Read the model definition and answer for the solid it produces. Units are mm, in the model's axes. A direction names the side the tool comes from. Coordinates: 2 decimals unless noted, no trailing zeros. Write each loop counter-clockwise with the first axis right and the second up, starting at its lowest first coordinate (ties: lowest second). Pieces come first, ordered by that corner, then holes.
1) Each of these flat-tipped pins is pushed along its axis until it touches: pin 1 Ø3 at (y, z) = (18.5, -111) entering from +X; pin 2 Ø4 at (y, z) = (13, -108) entering from -X; pin 3 Ø2 at (x, y) = (-32, 19) entering from -Z; pin 4 Ø5 at (x, z) = (-35.5, -108.5) entering from -Y. Where does it stop, or does it pass through?
2) Determine the mould class of faces 3 (the face through (-33.47, 0.246, -111.096)), 4 (the face through (-29.46, 0.74, -110.49)), 5 (the face through (-35, 1.5, -112)), 6 (the face through (-34.12, 11.87, -110.91)) for opening direction Z: +Z half, -Z half, draft (parallel to the pull), parting line (faces both ways), or undercut.
3) The part is cut by section A-A (y = 13). Determine the outline of the cut face in (x, z).
4) Find the intervals of material crossed by line 1 (Y direction, x = -30, z = -110.5); line 2 (Z direction, x = -34.25, y = 8.5); line 3 (Z direction, x = -32.75, y = 1.25), in increasing order.
5) Which of the six approach directions +Z, -Z, +X, -X, +Y, -Y give full straight-line access (tool end or side, diameter ignored) to faces 1 (the face through (-32.51, 0, -106.67)), 2 (the face through (-34, 0.5, -109))?
from build123d import *

# Parameters (mm, degrees)
SALIENTE_EXTRUIR1_DEPTH = 1.5
CROQUIS2_R              = 2.2
SALIENTE_EXTRUIR2_DEPTH = 20
FILLET2_R               = 1
SKETCH1_R               = 2.5
CUT_EXTRUDE1_DEPTH      = 0.5


with BuildPart() as part:
    # Croquis1 → Saliente-Extruir1 (new body)
    with BuildSketch(Plane(origin=(0, 0, 0), x_dir=(1, 0, 0), z_dir=(0, 1, 0))):
        with BuildLine():
            Line((-28.743638834, 108.856298042), (-28.28575881, 109.159080257))
            Line((-28.28575881, 109.159080257), (-30.66606326, 111.852582661))
            ThreePointArc((-30.66606326, 111.852582661), (-32.271190025, 113.035950486), (-34.220833362, 113.455095091))
            ThreePointArc((-34.220833362, 113.455095091), (-37.554900965, 105.336408582), (-29.477245058, 108.768689524))
            ThreePointArc((-29.477245058, 108.768689524), (-29.099722767, 108.722734742), (-28.743638834, 108.856298042))
        make_face()
    extrude(amount=SALIENTE_EXTRUIR1_DEPTH)

    # Croquis2 → Saliente-Extruir2 (add)
    with BuildSketch(Plane(origin=(0, 1.5, 0), x_dir=(1, 0, 0), z_dir=(0, 1, 0))):
        with Locations(Location((-34.220833362, 108.71115792, 0), (0, 0, 270))):
            Circle(CROQUIS2_R)
    extrude(amount=SALIENTE_EXTRUIR2_DEPTH)

    # Fillet2
    fillet2_edges = [part.edges().sort_by_distance(p)[0] for p in [
        (-34.220833362, 1.5, -110.91115792),
    ]]
    fillet(fillet2_edges, radius=FILLET2_R)

    # Sketch1 → Cut-Extrude1 (cut)
    with BuildSketch(Plane.XZ):
        with Locations(Location((-34.220833362, -108.71115792, 0), (0, 0, 270))):
            Circle(SKETCH1_R)
    extrude(amount=-CUT_EXTRUDE1_DEPTH, mode=Mode.SUBTRACT)


solid = part.part
Reported:
1. pin 1: stops at x = -32.17
1. pin 2: stops at x = -36.42
1. pin 3: stops at z = -110.54
1. pin 4: stops at y = 0
2. face 3: undercut
2. face 4: -Z half
2. face 5: draft
2. face 6: parting line
3. outline: circle Ø4.4 at (-34.22, -108.71)
4. line 1: y = 0 to 1.5
4. line 2: z = -110.91 to -106.51
4. line 3: z = -113.22 to -104.2
5. face 1: +Z, -Z, +X, -X, -Y
5. face 2: -Y
